For this review, use the dimensioned drawing (mm, ordinates from the lowest corner) and the shaded views. Round coordinates to 2 decimals unless told otherwise and drop trailing zeros. Order: outer loops, then holes, each group sorted by start corner. A loop starts at its lowest first (then second) coordinate and runs counter-clockwise, first axis right, second up. Notation, with made-up numbers: (50, 28) -> (95, 28) arc R18 cw to (95, 47) -> close; hole circle Ø11 at (-16, 18). An arc over 180 degrees is marked (long way). Answer in a Markdown table with one row per item.
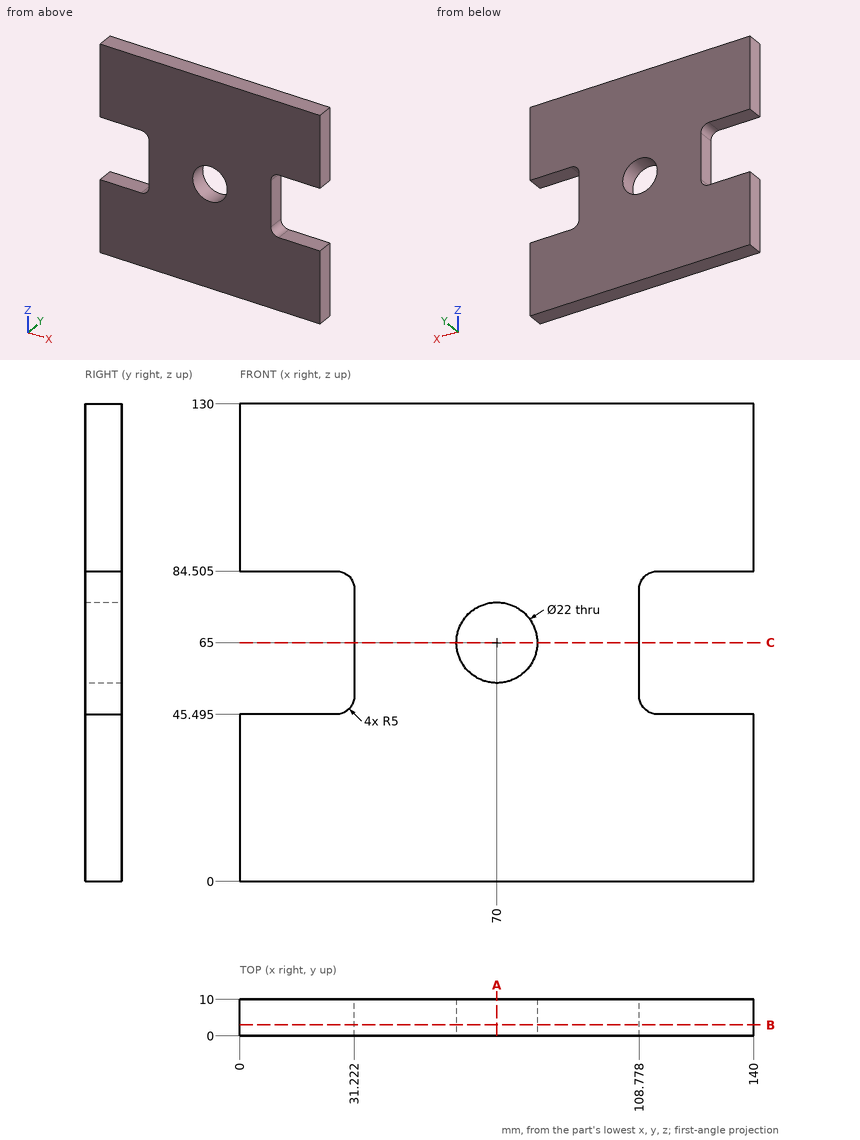
Q1. To check wall thickness, follow probe 1 along Z at (x, y) = (133, 4.5) (1 decimal); probe 2 along X at (y, z) = (7, 65); probe 3 along Z at (x, y) = (112.5, 8.25). State the ranges of each line that lie inside material, in increasing order.
Answer key:
| item | result |
|---|---|
| probe 1 | z = 0 to 45.5, 84.5 to 130 |
| probe 2 | x = 31.22 to 59, 81 to 108.78 |
| probe 3 | z = 0 to 45.66, 84.34 to 130 |
Q2. Clearance check with flat-ended pins moving along their axes: pin 1 Ø3 at (y, z) = (5, 70.5) entering from -X; pin 2 Ø3 at (y, z) = (1.5, 69.5) entering from +X. State where each tip first meets the part, or that it passes through.
Answer key:
| item | result |
|---|---|
| pin 1 | stops at x = 31.22 |
| pin 2 | stops at x = 108.78 |
Q3. Take a section at C-C, the plane z = 65. Write out the cut boundary in (x, y).
Answer key:
| item | result |
|---|---|
| outline | (31.22, 0) -> (59, 0) -> (59, 10) -> (31.22, 10) -> close; (81, 0) -> (108.78, 0) -> (108.78, 10) -> (81, 10) -> close |
Q4. Take a section at A-A, the plane x = 70. Write out the cut boundary in (y, z), then the cut area to 3 significant figures.
Answer key:
| item | result |
|---|---|
| outline | (0, 0) -> (10, 0) -> (10, 54) -> (0, 54) -> close; (0, 76) -> (10, 76) -> (10, 130) -> (0, 130) -> close |
| area | 1,080 mm^2 |
Q5. Take a section at B-B, the plane y = 3. Write out the cut boundary in (x, z) (1 decimal), then the cut area to 3 significant figures.
Answer key:
| item | result |
|---|---|
| outline | (0, 0) -> (140, 0) -> (140, 45.5) -> (113.8, 45.5) arc R5 cw to (108.8, 50.5) -> (108.8, 79.5) arc R5 cw to (113.8, 84.5) -> (140, 84.5) -> (140, 130) -> (0, 130) -> (0, 84.5) -> (26.2, 84.5) arc R5 cw to (31.2, 79.5) -> (31.2, 50.5) arc R5 cw to (26.2, 45.5) -> (0, 45.5) -> close; hole circle Ø22 at (70, 65) |
| area | 15,400 mm^2 |
